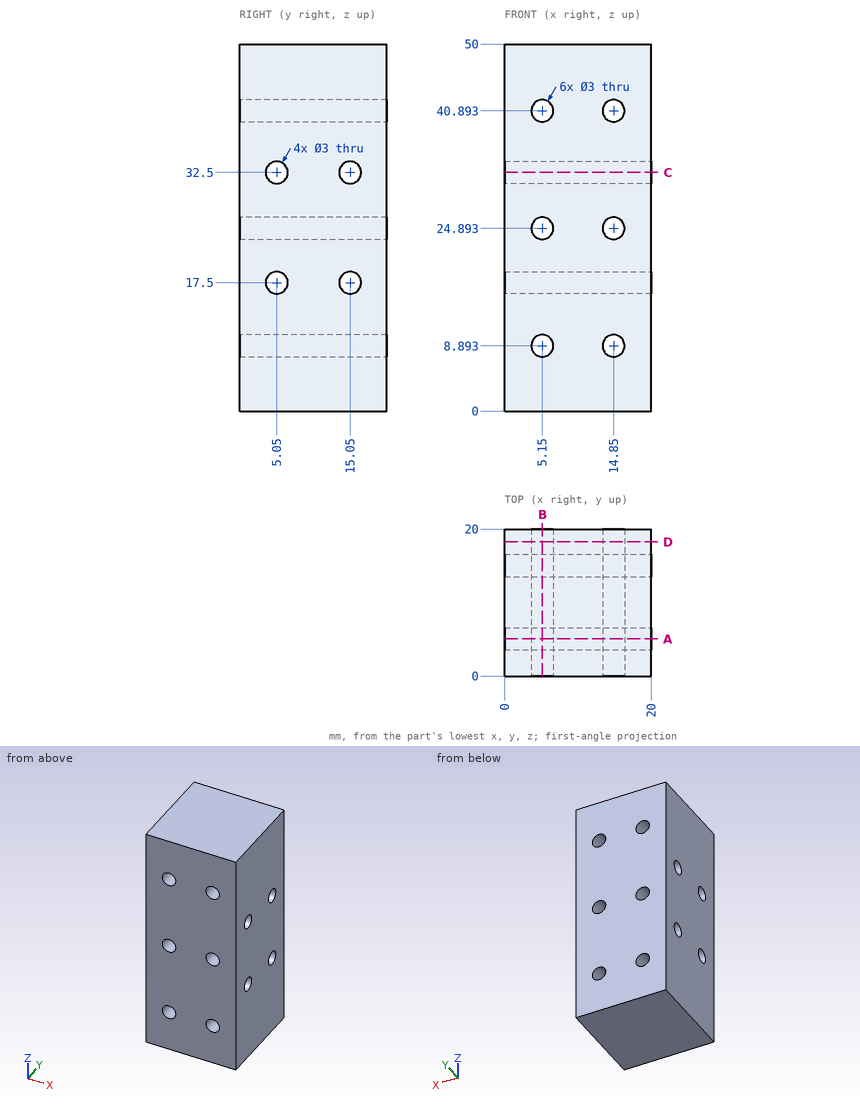
Job drawing, mm, ordinate dimensions from the low corner. One solid piece. Coordinates: 2 decimals unless noted, no trailing zeros. Write each loop counter-clockwise with the first axis right and the second up, starting at its lowest first coordinate (ties: lowest second). Pieces come first, ordered by that corner, then holes.
Item 1: Slice it at D-D (y = 18.25). Write the cut outline in (x, z).
Item 2: Slice it at A-A (y = 5.05). Count the separate pieces of the cut face and the enclosed holes in it, and give its area (3 significant figures).
Item 3: Probe line 1 (Y direction, x = 4.75, z = 17.5); line 2 (Z direction, x = 3.5, y = 15.5); line 3 (X direction, y = 15.75, z = 8). List the from-to ranges inside material, lowest first.
Item 4: Pin check, flat tip, straight feed: pin 1 (2.5 mm diameter, centred on x = 5.15, z = 40.89, fed in from +Y). Stop position of the tip, or through.
Item 5: Slice it at C-C (z = 32.5). Write the cut outline in (x, y).
Item 6: Slice it at B-B (x = 5.15). Write the cut outline in (y, z), and give its area (3 significant figures).
Results found:
1. outline: (0, 0) - (20, 0) - (20, 50) - (0, 50) - close; hole circle Ø3 at (5.15, 8.89); hole circle Ø3 at (5.15, 24.89); hole circle Ø3 at (5.15, 40.89); hole circle Ø3 at (14.85, 8.89); hole circle Ø3 at (14.85, 24.89); hole circle Ø3 at (14.85, 40.89)
2. separate pieces: 3
2. enclosed holes: 6
2. area: 838 mm2
3. line 1: y = 0 to 3.55, 6.55 to 13.55, 16.55 to 20
3. line 2: z = 0 to 16.07, 18.93 to 31.07, 33.93 to 50
3. line 3: x = 0 to 3.94, 6.36 to 13.64, 16.06 to 20
4. pin 1: passes through
5. outline: (0, 0) - (20, 0) - (20, 3.55) - (0, 3.55) - close; (0, 6.55) - (20, 6.55) - (20, 13.55) - (0, 13.55) - close; (0, 16.55) - (20, 16.55) - (20, 20) - (0, 20) - close
6. outline: (0, 0) - (20, 0) - (20, 7.39) - (0, 7.39) - close; (0, 10.39) - (20, 10.39) - (20, 23.39) - (0, 23.39) - close; (0, 26.39) - (20, 26.39) - (20, 39.39) - (0, 39.39) - close; (0, 42.39) - (20, 42.39) - (20, 50) - (0, 50) - close; hole circle Ø3 at (5.05, 17.5); hole circle Ø3 at (5.05, 32.5); hole circle Ø3 at (15.05, 17.5); hole circle Ø3 at (15.05, 32.5)
6. area: 792 mm2
